Here's how the part is built. I have some questions about the finished solid (model axes, mm). A direction names the side the tool comes from. Coordinates: 2 decimals unless noted, no trailing zeros. Loops run counter-clockwise (first coordinate to the right, second up) from the corner with the lowest first, then second, coordinate; pieces in that order, holes last. Notation, with made-up numbers: M -5,33 L 22,33 A11 cw 22,52 Z; hole C 52.5,11.25 d9. An arc over 180 degrees is marked long. Use CSV: the item, a comma, the result in double quotes. Start each with the question number.
Q1. If we section it at D-D (y = -2.5): Please give me the cut outline in (x, z), and give its area (3 significant figures).
Q2. If we section it at C-C (x = 6.75): Please give me the cut outline in (y, z).
Q3. For pin 1 Ø4 at (x, z) = (-5, 2.5) entering from +Y; pin 2 Ø8 at (x, y) = (6.5, 2) entering from -Z, each with a flat end and sliding along its axis, tell me the tip position at first contact or that it passes through.
Q4. If we section it at B-B (z = 5.5): Please give me the cut outline in (x, y), and give its area (3 significant figures).
Q5. If we mould it in two halves opening along Y, with no side actions, what happens to faces 1 (the cylindrical face through (0, 0, 7)), 2 (the flat face through (4, 8, 11)), 3 (the flat face through (4, -7.7, 9))? For each: +Y half, -Y half, draft (parallel to the pull), parting line (faces both ways), or undercut.
Q6. Which directions (+Z, -Z, +X, -X, +Y, -Y) give clear straight access to the entire face, cutting with the end or side of a thin tool? Please do faces 4 (the cylindrical face through (-8, 0, 6)), 5 (the flat face through (4, 7.7, 9)), 6 (the flat face through (-2, 0, 13)).
Q7. Please list where these lines run through material, in increasing order: probe 1 along Y at (x, z) = (2, 8.75); probe 2 along Y at (x, z) = (4.75, 11); probe 3 along Y at (x, z) = (-5.75, 5.25). Write a range as [from, to].
Q8. If we section it at A-A (x = 2): Please give me the cut outline in (y, z).
Autodesk Inventor part; units mm, degrees
ref_plane "YZ Plane" through (0, 0, 0) normal (1, 0, 0) x (0, 1, 0)
ref_plane "XZ Plane" through (0, 0, 0) normal (0, 1, 0) x (-1, 0, 0)
ref_plane "XY Plane" through (0, 0, 0) normal (0, 0, 1) x (1, 0, 0)
sketch "Sketch1" plane through (0, 0, 0) normal (0, 0, 1) x (1, 0, 0)
  circle A0 centre (0, 0) radius 8
  circle A1 centre (8, 0) radius 6 construction
  dimension "d0" = 16
  dimension "d1" = 12
extrude "Extrusion1" add sketch "Sketch1" along normal blind 13
sketch "Sketch2" plane through (0, 0, 13) normal (0, 0, 1) x (1, 0, 0)
  circle A0 centre (0, 0) radius 8
  circle A1 centre (8, 0) radius 8 construction
  line L0 (0, 8) -> (8, 8)
  line L1 (8, 8) -> (8, -8)
  line L2 (8, -8) -> (0, -8)
  line L3 (0, -8) -> (0, 8)
extrude "Extrusion2" add sketch "Sketch2" against normal blind 4 contours A0 L3 | L1 L2 A0 | A0 L0 L1 picked at (1.157, 2.4026)
sketch "Sketch3" plane through (0, 0, 13) normal (0, 0, 1) x (1, 0, 0)
  arc A0 (0, 8) -> (0, -8) centre (0, 0) ccw
  line L0 (8, 8) -> (8, -8)
  circle A1 centre (8, 0) radius 8
extrude "Extrusion3" cut sketch "Sketch3" against normal through all
properties part number "effector plug"
Results below:
1,outline,"M -7.6,0 L 0.4,0 L 0.4,13 L -7.6,13 Z"
1,area,"104 mm^2"
2,outline,"M -8,9 L -7.9,9 L -7.9,13 L -8,13 Z; M 7.9,9 L 8,9 L 8,13 L 7.9,13 Z"
3,pin 1,"y = 7.42"
3,pin 2,"through"
4,outline,"M 4,-6.93 A8 cw 4,6.93 A8 ccw long Z"
4,area,"122 mm^2"
5,face 1,"undercut"
5,face 2,"+Y half"
5,face 3,"draft"
6,face 4,"-Z"
6,face 5,"-Z, +X, +Y"
6,face 6,"+Z, +X, -X, +Y, -Y"
7,probe 1,"[-7.75, -5.29], [5.29, 7.75]"
7,probe 2,"[-8, -7.31], [7.31, 8]"
7,probe 3,"[-5.56, 5.56]"
8,outline,"M -8,9 L -7.75,9 L -7.75,0 L -5.29,0 L -5.29,13 L -8,13 Z; M 5.29,0 L 7.75,0 L 7.75,9 L 8,9 L 8,13 L 5.29,13 Z"
